from build123d import *

# Parameters (mm, degrees)
SKETCH1_W            = 101.6
SKETCH1_H            = 127
BOSS_EXTRUDE1_DEPTH  = 3.175
SKETCH2_W            = 101.6
SKETCH2_H            = 117.475
BOSS_EXTRUDE2_DEPTH  = 22.225
SKETCH3_W            = 88.9
SKETCH3_H            = 19.05
CUT_EXTRUDE1_DEPTH   = 3.175
SKETCH4_R            = 3.175
CUT_EXTRUDE2_DEPTH   = 165.150877625
SKETCH5_W            = 88.9
SKETCH5_H            = 6.477782688
CUT_EXTRUDE3_DEPTH   = 22.225
SKETCH6_W            = 88.9
SKETCH6_H            = 19.05
CUT_EXTRUDE4_DEPTH   = 3.175
SKETCH7_W            = 88.9
SKETCH7_H            = 88.9
CUT_EXTRUDE6_DEPTH   = 22.225
CUT_EXTRUDE7_DEPTH   = 7.62
LPATTERN1_COUNT      = 6
LPATTERN1_PITCH      = 12.7
SNAP_START           = 99.568
SNAP_GROOVE1_DEPTH   = 2.032
SNAP_START_2         = 97.536
SNAP_GROOVE1_2_DEPTH = 2.032
MIRROR2_START        = 99.568
MIRROR2_COPY_1_DEPTH = 2.032
MIRROR2_START_2      = 97.536
MIRROR2_COPY_2_DEPTH = 2.032
MIRROR2_COPY_3_DEPTH = 2.032
CUT_EXTRUDE8_REACH   = 157.023
LPATTERN2_COUNT      = 6
LPATTERN2_PITCH      = 12.7


# Read off the part's stored shape, not the designer's step: Snap Groove1
with BuildPart() as part:
    # Sketch1 → Boss-Extrude1 (new body)
    with BuildSketch(Plane.XY):
        with Locations((50.8, 63.5)):
            Rectangle(SKETCH1_W, SKETCH1_H)
    extrude(amount=BOSS_EXTRUDE1_DEPTH)

    # Sketch2 → Boss-Extrude2 (add)
    with BuildSketch(Plane.XY.offset(3.175)):
        with Locations((50.8, 58.7375)):
            Rectangle(SKETCH2_W, SKETCH2_H)
    extrude(amount=BOSS_EXTRUDE2_DEPTH)

    # Sketch3 → Cut-Extrude1 (cut)
    with BuildSketch(Plane(origin=(0, 117.475, 0), x_dir=(1, 0, 0), z_dir=(0, 1, 0))):
        with Locations((50.8, -12.7)):
            Rectangle(SKETCH3_W, SKETCH3_H)
    extrude(amount=-CUT_EXTRUDE1_DEPTH, mode=Mode.SUBTRACT)

    # Sketch4 → Cut-Extrude2 (cut, through all)
    with BuildSketch(Plane.XY.offset(3.175)):
        with Locations((25.4, 120.65)):
            Circle(SKETCH4_R)
        with Locations((76.2, 120.65)):
            Circle(SKETCH4_R)
    extrude(amount=-CUT_EXTRUDE2_DEPTH, mode=Mode.SUBTRACT)

    # Sketch5 → Cut-Extrude3 (cut)
    with BuildSketch(Plane.XY.offset(25.4)):
        with Locations((50.8, 9.588891344)):
            Rectangle(SKETCH5_W, SKETCH5_H)
    extrude(amount=-CUT_EXTRUDE3_DEPTH, mode=Mode.SUBTRACT)

    # Sketch6 → Cut-Extrude4 (cut)
    with BuildSketch(Plane(origin=(0, 6.35, 0), x_dir=(1, 0, 0), z_dir=(0, 1, 0))):
        with Locations((50.8, -12.7)):
            Rectangle(SKETCH6_W, SKETCH6_H)
    extrude(amount=-CUT_EXTRUDE4_DEPTH, mode=Mode.SUBTRACT)

    # Sketch7 → Cut-Extrude6 (cut)
    with BuildSketch(Plane.XY.offset(25.4)):
        with Locations((50.8, 63.627782688)):
            Rectangle(SKETCH7_W, SKETCH7_H)
    extrude(amount=-CUT_EXTRUDE6_DEPTH, mode=Mode.SUBTRACT)

    # Sketch9 → Cut-Extrude7 (cut)
    with BuildSketch(Plane(origin=(0, 19.177782688, 0), x_dir=(1, 0, 0), z_dir=(0, 1, 0))):
        with BuildLine():
            Line((15.875, -3.175), (22.225, -3.175))
            ThreePointArc((22.225, -3.175), (19.05, -6.35), (15.875, -3.175))
        make_face()
    cut_extrude7 = extrude(amount=-CUT_EXTRUDE7_DEPTH, mode=Mode.SUBTRACT)

    # LPattern1: Cut-Extrude7 ×6
    with Locations(*[(i * LPATTERN1_PITCH, 0, 0) for i in range(1, LPATTERN1_COUNT)]):
        add(cut_extrude7, mode=Mode.SUBTRACT)

    # Snap Groove1 outline → Snap Groove1 (cut)
    with BuildSketch(Plane.YZ.offset(SNAP_START)):
        Polygon((102.39375, 12.7), (103.059328797, 25.4), (89.028171203, 25.4), (89.69375, 12.7), align=None)
    snap_groove1 = extrude(amount=SNAP_GROOVE1_DEPTH, mode=Mode.SUBTRACT)

    # Snap Groove1 2 outline → Snap Groove1 2 (cut)
    with BuildSketch(Plane.YZ.offset(SNAP_START_2)):
        Polygon((102.39375, 12.7), (102.726539398, 19.05), (89.360960602, 19.05), (89.69375, 12.7), align=None)
    snap_groove1_2 = extrude(amount=SNAP_GROOVE1_2_DEPTH, mode=Mode.SUBTRACT)

    # Mirror1: Snap Groove1, Snap Groove1 2 across plane
    add(snap_groove1.mirror(Plane(origin=(50.8, 0, 0), x_dir=(0, 0, 1), z_dir=(1, 0, 0))), mode=Mode.SUBTRACT)
    add(snap_groove1_2.mirror(Plane(origin=(50.8, 0, 0), x_dir=(0, 0, 1), z_dir=(1, 0, 0))), mode=Mode.SUBTRACT)

    # Mirror2: Snap Groove1, Snap Groove1 2 across plane
    add(snap_groove1.mirror(Plane(origin=(0, 63.498392913, -0.319448634), x_dir=(0, 0.005030750815786494, 0.999987345693049), z_dir=(0, -0.9999873456930491, 0.0050307508157864935))), mode=Mode.SUBTRACT)
    add(snap_groove1_2.mirror(Plane(origin=(0, 63.498392913, -0.319448634), x_dir=(0, 0.005030750815786494, 0.999987345693049), z_dir=(0, -0.9999873456930491, 0.0050307508157864935))), mode=Mode.SUBTRACT)

    # Mirror2 copy 1 sketch → Mirror2 copy 1 (cut)
    with BuildSketch(Plane(origin=(101.6, 126.996785826, -0.638897269), x_dir=(0, -0.9999493830924595, 0.010061374310242954), z_dir=(-1, 0, 0)).offset(MIRROR2_START)):
        Polygon((102.39375, 12.7), (103.059328797, 25.4), (89.028171203, 25.4), (89.69375, 12.7), align=None)
    extrude(amount=MIRROR2_COPY_1_DEPTH, mode=Mode.SUBTRACT)

    # Mirror2 copy 2 sketch → Mirror2 copy 2 (cut)
    with BuildSketch(Plane(origin=(101.6, 126.996785826, -0.638897269), x_dir=(0, -0.9999493830924595, 0.010061374310242954), z_dir=(-1, 0, 0)).offset(MIRROR2_START_2)):
        Polygon((102.39375, 12.7), (102.726539398, 19.05), (89.360960602, 19.05), (89.69375, 12.7), align=None)
    extrude(amount=MIRROR2_COPY_2_DEPTH, mode=Mode.SUBTRACT)

    # Mirror2 copy 3 sketch → Mirror2 copy 3 (cut)
    with BuildSketch(Plane(origin=(0, 126.996785826, -0.638897269), x_dir=(0, -0.9999493830924595, 0.010061374310242954), z_dir=(1, 0, 0)).offset(MIRROR2_START_2)):
        Polygon((102.39375, -12.7), (102.726539398, -19.05), (89.360960602, -19.05), (89.69375, -12.7), align=None)
    extrude(amount=MIRROR2_COPY_3_DEPTH, mode=Mode.SUBTRACT)

    # Sketch11 → Cut-Extrude8 (cut, up to next)
    with BuildSketch(Plane(origin=(0, 114.3, 0), x_dir=(1, 0, 0), z_dir=(0, 1, 0)), mode=Mode.PRIVATE) as cut_extrude8_sk1:
        with BuildLine():
            Line((15.875, -3.175), (22.225, -3.175))
            ThreePointArc((22.225, -3.175), (19.05, -6.35), (15.875, -3.175))
        make_face()
    cut_extrude8_tool1 = extrude(cut_extrude8_sk1.sketch, amount=-CUT_EXTRUDE8_REACH, mode=Mode.PRIVATE) & part.part
    cut_extrude8 = cut_extrude8_tool1.solids().sort_by_distance((19.05, 114.3, 4.522512))[0]
    add(cut_extrude8, mode=Mode.SUBTRACT)

    # LPattern2: Cut-Extrude8 ×6
    with Locations(*[(i * LPATTERN2_PITCH, 0, 0) for i in range(1, LPATTERN2_COUNT)]):
        add(cut_extrude8, mode=Mode.SUBTRACT)


solid = part.part
Model file for the job. Use its own axes, mm. A direction names the side the tool comes from. Give positions to 0.01 mm unless a question says otherwise; leave off trailing zeros. Order: outer loops, then holes, each group sorted by start corner. A loop starts at its lowest first (then second) coordinate and runs counter-clockwise, first axis right, second up. Notation, with made-up numbers: (48, 85.5) -> (72, 85.5) arc R23 ccw to (72, 104.5) -> close; hole circle Ø3 at (-30, 36.5). An arc over 180 degrees is marked (long way). Use CSV: the item, a comma, the result in double quotes.
1. Drill centre lines: line 1 along Y through (x, z) = (12, 17.5) (3 decimals); line 2 along Y through (x, z) = (58.5, 23) (3 decimals); line 3 along X through (y, z) = (38, 4.5). Where is each one in solid material? Low to high. Write a range as from..to.
Outcome:
line 1,"0..3.175, 12.828..19.178, 108.078..114.3"
line 2,"0..6.35, 12.828..19.178, 108.078..117.475"
line 3,"0..6.35, 95.25..101.6"
2. Band-saw the part on C-C, the plane x = 25.4. Give the cut face in (y, z) (3 decimals), then the cut area to 3 significant figures.
Outcome:
outline,"(0, 0) -> (117.475, 0) -> (117.475, 3.175) -> (114.3, 3.175) -> (114.3, 22.225) -> (117.475, 22.225) -> (117.475, 25.4) -> (108.078, 25.4) -> (108.078, 3.175) -> (19.178, 3.175) -> (19.178, 25.4) -> (12.828, 25.4) -> (12.828, 3.175) -> (3.175, 3.175) -> (3.175, 22.225) -> (6.35, 22.225) -> (6.35, 25.4) -> (0, 25.4) -> close; (123.825, 0) -> (127, 0) -> (127, 3.175) -> (123.825, 3.175) -> close"
area,"753 mm²"
3. Band-saw the part on D-D, the plane y = 40. Give the cut face in (x, z) (3 decimals).
Outcome:
outline,"(0, 0) -> (101.6, 0) -> (101.6, 25.4) -> (95.25, 25.4) -> (95.25, 3.175) -> (6.35, 3.175) -> (6.35, 25.4) -> (0, 25.4) -> close"
4. Band-saw the part on B-B, the plane y = 120.65. Give the cut face in (x, z) (3 decimals).
Outcome:
outline,"(0, 0) -> (22.225, 0) -> (22.225, 3.175) -> (0, 3.175) -> close; (28.575, 0) -> (73.025, 0) -> (73.025, 3.175) -> (28.575, 3.175) -> close; (79.375, 0) -> (101.6, 0) -> (101.6, 3.175) -> (79.375, 3.175) -> close"
5. Drop flat-ended pins along their axis: pin 1 (4 mm diameter, centred on x = 53, y = 31, fed in from +Z) (3 decimals); pin 2 (3 mm diameter, centred on y = 33.5, z = 23.5, fed in from -X); pin 3 (1.9 mm diameter, centred on y = 33, z = 16.5, fed in from +X). Give the stop position or say it passes through.
Outcome:
pin 1,"z = 3.175"
pin 2,"x = 2.03"
pin 3,"x = 97.54"
6. Band-saw the part on A-A, the plane x = 69.85. Give the cut face in (y, z) (3 decimals), then the cut area to 3 significant figures.
Outcome:
outline,"(0, 0) -> (127, 0) -> (127, 3.175) -> (3.175, 3.175) -> (3.175, 22.225) -> (6.35, 22.225) -> (6.35, 25.4) -> (0, 25.4) -> close; (12.828, 6.35) -> (19.178, 6.35) -> (19.178, 25.4) -> (12.828, 25.4) -> close; (108.078, 6.35) -> (114.3, 6.35) -> (114.3, 22.225) -> (117.475, 22.225) -> (117.475, 25.4) -> (108.078, 25.4) -> close"
area,"733 mm²"
7. Mould opens along Y. For faces 1 (the cylindrical face through (31.82, 111.23, 6.35)), 2 (the flat face through (2.032, 31, 22)) say: +Y half, -Y half, draft (parallel to the pull), parting line (faces both ways), or undercut.
Outcome:
face 1,"draft"
face 2,"undercut"
8. 3-axis set-ups, long thin cutter, end or side, ignore diameter. For faces 3 (the flat face through (50, 3.175, 13)), 4 (the flat face through (4.064, 31, 16)), 5 (the flat face through (6.35, 63, 14)): which of +Z, -Z, +X, -X, +Y, -Y reach the whole face in a straight line?
Outcome:
face 3,"none"
face 4,"-X"
face 5,"+Z"
